Source: CAD feature listing. Evaluate the final solid. Frame: model axes, mm. Give positions to 0.01 mm unless a question says otherwise; leave off trailing zeros. Answer as a JSON object with one key per item and string values. Group by question number.
Autodesk Inventor part; units mm, degrees
ref_plane "YZ Plane" through (0, 0, 0) normal (1, 0, 0) x (0, 1, 0)
ref_plane "XZ Plane" through (0, 0, 0) normal (0, 1, 0) x (-1, 0, 0)
sketch "layer_layout_sketch" plane through (0, 0, 0) normal (0, 0, 1) x (1, 0, 0)
  line L0 (-400, 200) -> (400, 200)
  line L1 (400, 200) -> (400, -200)
  line L2 (400, -200) -> (-400, -200)
  line L3 (-400, -200) -> (-400, 200)
  line L4 (0, 200) -> (0, -200) construction
  point P0 (0, 0)
  point P1 (0, 0)
  dimension "d116" = 400
  dimension "d117" = 800
sketch "coil_layer_sketch_lower" plane through (0, 0, 0) normal (0, 0, 1) x (1, 0, 0)
  line L0 (0, -9.3) -> (376.5, -9.3)
  line L1 (395, -27.8) -> (395, -131.5)
  line L2 (376.5, -150) -> (-376.5, -150)
  line L3 (-395, -131.5) -> (-395, -50.9)
  line L4 (0, -9.3) -> (0, -13.8)
  line L5 (0, -13.8) -> (375.5, -13.8)
  line L6 (390.5, -28.8) -> (390.5, -130.5)
  line L7 (375.5, -145.5) -> (-375.5, -145.5)
  line L8 (-376.5, -32.4) -> (363.75, -32.4)
  line L9 (382.25, -50.9) -> (382.25, -118.75)
  line L10 (363.75, -137.25) -> (-363.75, -137.25)
  line L11 (-390.5, -130.5) -> (-390.5, -51.9)
  line L12 (-375.5, -36.9) -> (362.75, -36.9)
  line L13 (377.75, -51.9) -> (377.75, -117.75)
  line L14 (362.75, -132.75) -> (-362.75, -132.75)
  line L15 (-377.75, -117.75) -> (-377.75, -75)
  line L16 (-382.25, -118.75) -> (-382.25, -74)
  line L17 (-363.75, -55.5) -> (351, -55.5)
  line L18 (369.5, -74) -> (369.5, -106)
  line L19 (-362.75, -60) -> (350, -60)
  line L20 (365, -75) -> (365, -105)
  line L21 (-558.3641, 0) -> (558.3641, 0)
  line L22 (350, -120) -> (-350, -120)
  line L23 (351, -124.5) -> (-351, -124.5)
  line L24 (-369.5, -106) -> (-369.5, -71.7563)
  line L25 (-369.5, -71.7563) -> (-365, -71.7563)
  line L26 (-365, -71.7563) -> (-365, -105)
  arc A0 (395, -27.8) -> (376.5, -9.3) centre (376.5, -27.8) ccw
  arc A1 (382.25, -50.9) -> (363.75, -32.4) centre (363.75, -50.9) ccw
  arc A2 (369.5, -74) -> (351, -55.5) centre (351, -74) ccw
  arc A3 (351, -124.5) -> (369.5, -106) centre (351, -106) ccw
  arc A4 (363.75, -137.25) -> (382.25, -118.75) centre (363.75, -118.75) ccw
  arc A5 (376.5, -150) -> (395, -131.5) centre (376.5, -131.5) ccw
  arc A6 (-395, -131.5) -> (-376.5, -150) centre (-376.5, -131.5) ccw
  arc A7 (-382.25, -118.75) -> (-363.75, -137.25) centre (-363.75, -118.75) ccw
  arc A8 (-369.5, -106) -> (-351, -124.5) centre (-351, -106) ccw
  arc A9 (-376.5, -32.4) -> (-395, -50.9) centre (-376.5, -50.9) ccw
  arc A10 (-363.75, -55.5) -> (-382.25, -74) centre (-363.75, -74) ccw
  arc A11 (-375.5, -36.9) -> (-390.5, -51.9) centre (-375.5, -51.9) ccw
  arc A12 (-362.75, -60) -> (-377.75, -75) centre (-362.75, -75) ccw
  arc A13 (-390.5, -130.5) -> (-375.5, -145.5) centre (-375.5, -130.5) ccw
  arc A14 (-377.75, -117.75) -> (-362.75, -132.75) centre (-362.75, -117.75) ccw
  arc A15 (-365, -105) -> (-350, -120) centre (-350, -105) ccw
  arc A16 (350, -120) -> (365, -105) centre (350, -105) ccw
  arc A17 (362.75, -132.75) -> (377.75, -117.75) centre (362.75, -117.75) ccw
  arc A18 (375.5, -145.5) -> (390.5, -130.5) centre (375.5, -130.5) ccw
  arc A19 (377.75, -51.9) -> (362.75, -36.9) centre (362.75, -51.9) ccw
  arc A20 (390.5, -28.8) -> (375.5, -13.8) centre (375.5, -28.8) ccw
  arc A21 (365, -75) -> (350, -60) centre (350, -75) ccw
  point P0 (0, 0)
  point P1 (0, 0)
  point P2 (368.0934, -60)
  point P3 (370, -61.9066)
  point P4 (0, -150)
  dimension "d1" = 4.5
  dimension "d2" = 4.5
  dimension "d3" = 4.5
  dimension "d4" = 9.3
  dimension "d5" = 790
  dimension "d6" = 395
  dimension "d7" = 4.5
  dimension "d8" = 4.5
  dimension "d9" = 8.25
  dimension "d10" = 4.5
  dimension "d11" = 18.6
  dimension "d12" = 4.5
  dimension "d13" = 8.25
  dimension "d14" = 4.5
  dimension "d15" = 4.5
  dimension "d16" = 4.5
  dimension "d17" = 8.25
  dimension "d19" = 18.6
  dimension "d20" = 8.25
  dimension "d82" = 150
  dimension "d88" = 4.5
  dimension "d89" = 8.25
  dimension "d96" = 4.5
  dimension "d97" = 8.25
  dimension "d98" = 18.5
  dimension "d99" = 15
  dimension "d109" = 15
sketch "coil_layer_sketch_upper" plane through (0, 0, 0) normal (0, 0, 1) x (1, 0, 0)
  line L0 (0, -13.8) -> (-376.5, -13.8)
  line L1 (-395, 4.7) -> (-395, 131.5)
  line L2 (-376.5, 150) -> (376.5, 150)
  line L3 (395, 131.5) -> (395, 27.8)
  line L4 (0, -9.3) -> (-375.5, -9.3)
  line L5 (-390.5, 5.7) -> (-390.5, 130.5)
  line L6 (-375.5, 145.5) -> (375.5, 145.5)
  line L7 (390.5, 130.5) -> (390.5, 28.8)
  line L8 (375.5, 13.8) -> (-362.75, 13.8)
  line L9 (-377.75, 28.8) -> (-377.75, 117.75)
  line L10 (376.5, 9.3) -> (-363.75, 9.3)
  line L11 (-382.25, 27.8) -> (-382.25, 118.75)
  line L12 (-362.75, 132.75) -> (362.75, 132.75)
  line L13 (-363.75, 137.25) -> (363.75, 137.25)
  line L14 (377.75, 117.75) -> (377.75, 51.9)
  line L15 (362.75, 36.9) -> (-350, 36.9)
  line L16 (382.25, 118.75) -> (382.25, 50.9)
  line L17 (363.75, 32.4) -> (-351, 32.4)
  line L18 (-365, 51.9) -> (-365, 105)
  line L19 (-350, 120) -> (350, 120)
  line L20 (365, 105) -> (365, 75)
  line L21 (350, 60) -> (-356.75, 60)
  line L22 (-369.5, 50.9) -> (-369.5, 106)
  line L23 (-351, 124.5) -> (351, 124.5)
  line L24 (369.5, 106) -> (369.5, 74)
  line L25 (351, 55.5) -> (-356.75, 55.5)
  line L26 (-356.75, 60) -> (-356.75, 55.5)
  line L27 (-700, 0) -> (700, 0)
  line L28 (-980, 0) -> (980, 0)
  line L29 (0, -13.8) -> (0, -9.3)
  line L30 (0, -51.9241) -> (0, 188.1241)
  arc A0 (365, 105) -> (350, 120) centre (350, 105) ccw
  arc A1 (350, 60) -> (365, 75) centre (350, 75) ccw
  arc A2 (377.75, 117.75) -> (362.75, 132.75) centre (362.75, 117.75) ccw
  arc A3 (362.75, 36.9) -> (377.75, 51.9) centre (362.75, 51.9) ccw
  arc A4 (390.5, 130.5) -> (375.5, 145.5) centre (375.5, 130.5) ccw
  arc A5 (375.5, 13.8) -> (390.5, 28.8) centre (375.5, 28.8) ccw
  arc A6 (-350, 120) -> (-365, 105) centre (-350, 105) ccw
  arc A7 (-365, 51.9) -> (-350, 36.9) centre (-350, 51.9) ccw
  arc A8 (-377.75, 28.8) -> (-362.75, 13.8) centre (-362.75, 28.8) ccw
  arc A9 (-390.5, 5.7) -> (-375.5, -9.3) centre (-375.5, 5.7) ccw
  arc A10 (-362.75, 132.75) -> (-377.75, 117.75) centre (-362.75, 117.75) ccw
  arc A11 (-375.5, 145.5) -> (-390.5, 130.5) centre (-375.5, 130.5) ccw
  arc A12 (-376.5, 150) -> (-395, 131.5) centre (-376.5, 131.5) ccw
  arc A13 (-363.75, 137.25) -> (-382.25, 118.75) centre (-363.75, 118.75) ccw
  arc A14 (-351, 124.5) -> (-369.5, 106) centre (-351, 106) ccw
  arc A15 (-369.5, 50.9) -> (-351, 32.4) centre (-351, 50.9) ccw
  arc A16 (-382.25, 27.8) -> (-363.75, 9.3) centre (-363.75, 27.8) ccw
  arc A17 (-395, 4.7) -> (-376.5, -13.8) centre (-376.5, 4.7) ccw
  arc A18 (351, 55.5) -> (369.5, 74) centre (351, 74) ccw
  arc A19 (363.75, 32.4) -> (382.25, 50.9) centre (363.75, 50.9) ccw
  arc A20 (376.5, 9.3) -> (395, 27.8) centre (376.5, 27.8) ccw
  arc A21 (395, 131.5) -> (376.5, 150) centre (376.5, 131.5) ccw
  arc A22 (382.25, 118.75) -> (363.75, 137.25) centre (363.75, 118.75) ccw
  arc A23 (369.5, 106) -> (351, 124.5) centre (351, 106) ccw
  point P0 (0, 0)
  point P1 (395, 9.3)
  point P2 (-382.25, 9.3)
  point P3 (0, 150)
  point P4 (-700, 0)
  point P5 (700, 0)
  point P6 (0, 150)
  dimension "d58" = 4.5
  dimension "d59" = 4.5
  dimension "d60" = 4.5
  dimension "d61" = 8.25
  dimension "d62" = 8.25
  dimension "d64" = 4.5
  dimension "d65" = 4.5
  dimension "d66" = 4.5
  dimension "d67" = 8.25
  dimension "d69" = 18.6
  dimension "d70" = 4.5
  dimension "d71" = 4.5
  dimension "d72" = 18.6
  dimension "d73" = 8.25
  dimension "d74" = 8.25
  dimension "d75" = 4.5
  dimension "d77" = 18.6
  dimension "d78" = 4.5
  dimension "d79" = 4.5
  dimension "d80" = 4.5
  dimension "d83" = 150
  dimension "d87" = 8.25
  dimension "d91" = 4.5
  dimension "d92" = 9.3
  dimension "d93" = 790
  dimension "d100" = 15
  dimension "d101" = 18.5
  dimension "d102" = 8.25
extrude "layer_sheet Extrude" add sketch "layer_layout_sketch" along normal blind 4.5
extrude "wire_holes_upper Cut" cut sketch "coil_layer_sketch_upper" along normal blind 4.5 contours L0 A17 L27 A9 L4 L29 | A17 L1 A12 L2 L30 L6 A11 L5 A9 L27 | L30 L8 A5 L7 A4 L6 L2 A21 L3 A20 L10 | L10 A16 L11 A13 L13 L30 L12 A10 L9 A8 L8 | L30 L15 A3 L14 A2 L12 L13 A22 L16 A19 L17 | L17 A15 L22 A14 L23 L30 L19 A6 L18 A7 L15 | L30 L21 A1 L20 A0 L19 L23 A23 L24 A18 L25 | L25 L26 L21 L30
extrude "wire_holes_lower Cut" cut sketch "coil_layer_sketch_lower" along normal blind 4.5
equation "\"d1\" = wire_diameter"
equation "\"d2\" = wire_diameter"
equation "\"d3\" = wire_diameter"
equation "\"d4\" = 0.5 * distance_between_wires"
equation "\"d7\" = wire_diameter"
equation "\"d8\" = wire_diameter"
equation "\"d9\" = distance_between_wires_edge"
equation "\"d10\" = wire_diameter"
equation "\"d11\" = distance_between_wires"
equation "\"d12\" = wire_diameter"
equation "\"d13\" = distance_between_wires_edge"
equation "\"d14\" = wire_diameter"
equation "\"d15\" = wire_diameter"
equation "\"d16\" = wire_diameter"
equation "\"d17\" = distance_between_wires_edge"
equation "\"d19\" = distance_between_wires"
equation "\"d20\" = distance_between_wires_edge"
equation "\"d82\" = 0.5 * track_width"
equation "\"d58\" = wire_diameter"
equation "\"d59\" = wire_diameter"
equation "\"d60\" = wire_diameter"
equation "\"d61\" = distance_between_wires_edge"
equation "\"d62\" = distance_between_wires_edge"
equation "\"d64\" = wire_diameter"
equation "\"d65\" = wire_diameter"
equation "\"d66\" = wire_diameter"
equation "\"d67\" = distance_between_wires_edge"
equation "\"d69\" = distance_between_wires"
equation "\"d70\" = wire_diameter"
equation "\"d71\" = wire_diameter"
equation "\"d72\" = distance_between_wires"
equation "\"d73\" = distance_between_wires_edge"
equation "\"d74\" = distance_between_wires_edge"
equation "\"d75\" = wire_diameter"
equation "\"d77\" = distance_between_wires"
equation "\"d78\" = wire_diameter"
equation "\"d79\" = wire_diameter"
equation "\"d80\" = wire_diameter"
equation "\"d83\" = 0.5 * track_width"
equation "\"wire_diameter\" = 4.5"
equation "\"distance_between_wires\" = -1.2 * wire_diameter + 0.2 * parameter_6"
equation "\"distance_between_wires_edge\" = 8.25"
equation "\"bend_radius_inner\" = 15"
equation "\"bend_radius_outer\" = 18.5"
properties part number "primary_coil_0R2"
Q1. First-contact query: pin 1 Ø8 at (x, y) = (125.5, -96.5) entering from -Z. Flat tip, straight axial feed; report the tip coordinate or a pass-through.
Q2. Section A-A on x = 180. State how many separate pieces and enclosed holes the cut face has, then the cut area to 3 significant figures.
Q3. Ray query, probe 1 along X at (y, z) = (-140, 1.45); probe 2 along X at (y, z) = (-30, 3.05); probe 3 along X at (y, z) = (-7, 0.95). Return the intervals inside material, ascending. Write a range as [from, to].
Taken from the geometry:
{
 "1": {"pin 1": "stops at z = 0"},
 "2": {"separate pieces": "13", "enclosed holes": "0", "area": "1,560 mm²"},
 "3": {"probe 1": "x = [-400, -392.93], [-387.11, 387.11], [392.93, 400]", "probe 2": "x = [-400, 390.5], [395, 400]", "probe 3": "x = [-400, -390.83], [-383.48, 400]"}
}
